The listing builds one solid part. Answer for the finished solid, in the listing's coordinates (mm). Face numbers are marked on the shaded views. Round coordinates to 2 decimals unless told otherwise and drop trailing zeros. Loops run counter-clockwise (first coordinate to the right, second up) from the corner with the lowest first, then second, coordinate; pieces in that order, holes last. Notation, with made-up numbers: M -6,4.25 L 12,4.25 A31 cw 12,42.25 Z; hole C 20,-0.5 d9. An arc over 180 degrees is marked long. Answer as a JSON object with one key per item and string values.
```python
from build123d import *

# Parameters (mm, degrees)
SKETCH_R        = 77.5
PAD_DEPTH       = 25
FILLET_R        = 3
SKETCH001_R     = 65
POCKET_DEPTH    = 20
SKETCH002_W     = 5
SKETCH002_H     = 20
POCKET001_DEPTH = 15
FILLET001_R     = 3


with BuildPart() as part:
    # Sketch → Pad (new body)
    with BuildSketch(Plane.XY):
        Circle(SKETCH_R)
    extrude(amount=PAD_DEPTH)

    # Fillet
    fillet_edges = [part.edges().sort_by_distance(p)[0] for p in [
        (-77.5, 0, 25),
    ]]
    fillet(fillet_edges, radius=FILLET_R)

    # Sketch001 → Pocket (cut)
    with BuildSketch(Plane.XY):
        Circle(SKETCH001_R)
    extrude(amount=POCKET_DEPTH, mode=Mode.SUBTRACT)

    # Sketch002 → Pocket001 (cut)
    with BuildSketch(Plane.XZ.offset(78)):
        with Locations((0, 10)):
            Rectangle(SKETCH002_W, SKETCH002_H)
    extrude(amount=-POCKET001_DEPTH, mode=Mode.SUBTRACT)

    # Fillet001
    fillet001_edges = [part.edges().sort_by_distance(p)[0] for p in [
        (55.677644, -53.909647, 0),
        (-53.909647, 55.677644, 0),
    ]]
    fillet(fillet001_edges, radius=FILLET001_R)


solid = part.part
```
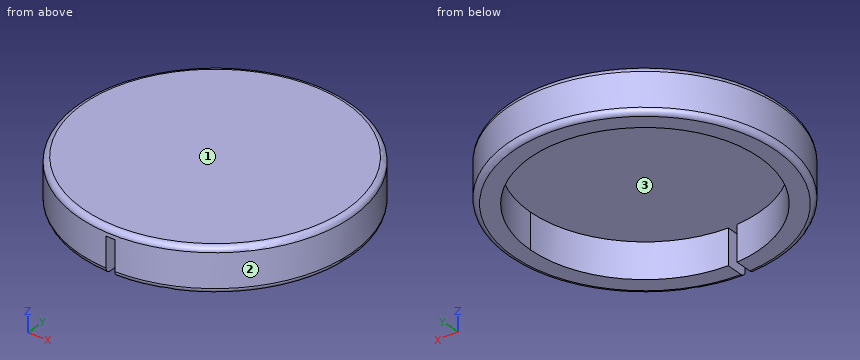
Item 1: Straight lines are drawn through the part: line 1 (X direction, y = 0, z = 11); line 2 (Y direction, x = 0, z = 11.5); line 3 (Y direction, x = -16, z = 6.75). For each, find the intervals that lie inside material, in ascending order.
Values follow:
{"line 1": "-77.5 to -65, 65 to 77.5", "line 2": "65 to 77.5", "line 3": "-75.83 to -63, 63 to 75.83"}
Item 2: Flat-ended cylindrical pins translate along their axes: P1, Ø2, axis at x = -38.5, z = 22, coming from the +Y side; P2, Ø4, axis at x = 45.5, y = 47, coming from the -Z side; P3, Ø14, axis at y = -70, z = 9, coming from the -X side; P4, Ø6, axis at x = -30.5, y = -43.5, coming from the -Z side. Find the tip coordinate at first contact, or state that the pin passes through.
Values follow:
{"P1": "y = 67.82", "P2": "z = 0", "P3": "x = -45.14", "P4": "z = 20"}
Item 3: The part is cut by section A-A (x = 0). Give the vertices of the cut face in (y, z), then the cut area to 3 significant figures.
Values follow:
{"outline": "M -77.5,20 L 65,20 L 65,0 L 74.5,0 A3 ccw 77.5,3 L 77.5,22 A3 ccw 74.5,25 L -74.5,25 A3 ccw -77.5,22 Z", "area": "1,020 mm^2"}
Item 4: The part is cut by section B-B (z = 15.5). Give the vertices of the cut face in (x, y).
Values follow:
{"outline": "M -2.5,-77.46 L -2.5,-64.95 A65 cw long 2.5,-64.95 L 2.5,-77.46 A77.5 ccw long Z"}
Item 5: Determine the mould class of the marked faces 1, 2 and 3 for opening direction Y: released by +Y, released by -Y, zero draft, split by the parting line, or undercut.
Values follow:
{"face 1": "zero draft", "face 2": "split by the parting line", "face 3": "undercut"}
